Design review of the part built by this model. Coordinates are the model's own, in mm. Face numbers are marked on the shaded views. Round coordinates to 2 decimals unless told otherwise and drop trailing zeros. Loops run counter-clockwise (first coordinate to the right, second up) from the corner with the lowest first, then second, coordinate; pieces in that order, holes last. Notation, with made-up numbers: M 26.25,-7 L 43.25,-7 A30 ccw 43.25,26 Z; hole C 32.5,20 d9. An arc over 180 degrees is marked long. One line per item, written item: value. Start each with the question number.
Item 1: We need section A-A (y = 0). Write out the cut boundary in (x, z) (3 decimals).
Item 2: Clearance check with flat-ended pins moving along their axes: pin 1 (2 mm diameter, centred on x = 30.5, y = 19, fed in from +Z); pin 2 (2 mm diameter, centred on y = -53.5, z = 3, fed in from -X); pin 3 (10 mm diameter, centred on x = -39, z = 21, fed in from -Y). State where each tip first meets the part, or that it passes through.
Item 3: Mouldability with a two-part tool opening along Y and no side actions: class the marked faces 1, 2 and 3 as released by +Y, released by -Y, zero draft, split by the parting line, or undercut.
Item 4: For line 1 along Y through (x, z) = (0, 19.25) (3 decimals); line 2 along Z through (x, y) = (-48.5, -41.5); line 3 along X through (y, z) = (62, 14), list the stretches that pass through material, from the lowest coordinate up.
Item 5: We need section C-C (z = 20.75). Write out the cut boundary in (x, y) (3 decimals).
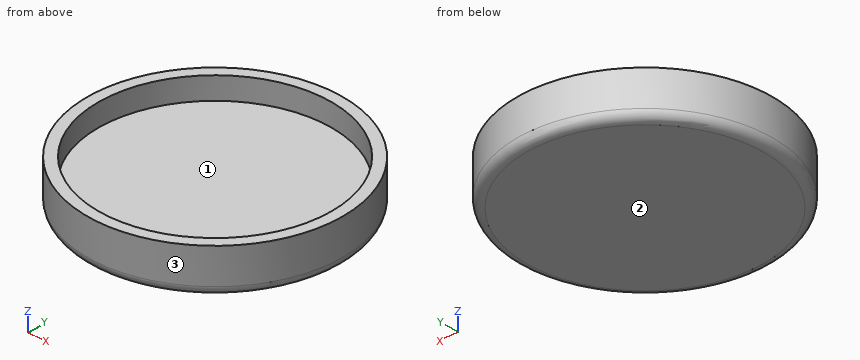
from build123d import *

# Parameters (mm, degrees)
F0_R     = 73.025
F0_R_2   = 66.675
F1_DEPTH = 25.4
F2_R     = 66.675
F3_DEPTH = 12.7
F4_R     = 5.08


with BuildPart() as f1:
    # F0 (on Top) → F1 (new body)
    with BuildSketch(Plane.XY):
        Circle(F0_R)
        Circle(F0_R_2, mode=Mode.SUBTRACT)
    extrude(amount=F1_DEPTH)

    # F2 (on Top) → F3 (join)
    with BuildSketch(Plane.XY):
        Circle(F2_R)
    extrude(amount=F3_DEPTH)

    # F4
    f4_edges = [f1.edges().sort_by_distance(p)[0] for p in [
        (-73.025, 0, 0),
    ]]
    fillet(f4_edges, radius=F4_R)


solid = f1.part
A:
1. outline: M -73.025,5.08 A5.08 ccw -67.945,0 L 67.945,0 A5.08 ccw 73.025,5.08 L 73.025,25.4 L 66.675,25.4 L 66.675,12.7 L -66.675,12.7 L -66.675,25.4 L -73.025,25.4 Z
2. pin 1: z = 12.7
2. pin 2: x = -50.26
2. pin 3: y = -64.63
3. face 1: undercut
3. face 2: zero draft
3. face 3: split by the parting line
4. line 1: -73.025 to -66.675, 66.675 to 73.025
4. line 2: 0 to 12.7
4. line 3: -38.58 to -24.53, 24.53 to 38.58
5. outline: C 0,0 d146.05; hole C 0,0 d133.35
